```python
from build123d import *

# Parameters (mm, degrees)
F0_R     = 3.175
F1_DEPTH = 57.5
F2_R     = 5
F2_R_2   = 3.175
F3_DEPTH = 5
F4_R     = 4.99999


# Not quite as in the source:
# - a fillet or chamfer is up to 0.001 mm smaller than in the source, because OpenCascade refuses the exact size


with BuildPart() as f1:
    # F0 (on Top) → F1 (new body)
    with BuildSketch(Plane.XY):
        Circle(F0_R)
    extrude(amount=F1_DEPTH)

    # F2 (on face) → F3 (join)
    with BuildSketch(Plane.XY.offset(57.5)):
        Circle(F2_R)
        Circle(F2_R_2, mode=Mode.SUBTRACT)
        Circle(F2_R_2)
    extrude(amount=F3_DEPTH)

    # F4 (radius 5 in the source; OpenCascade refuses exactly that, so slightly less here)
    f4_edges = [f1.edges().sort_by_distance(p)[0] for p in [
        (-5, 0, 62.5),
    ]]
    fillet(f4_edges, radius=F4_R)


solid = f1.part
```
Can you work these out from the model? Positions are in its coordinate system, mm. A direction names the side the tool comes from. Coordinates: 2 decimals unless noted, no trailing zeros. Write each loop counter-clockwise with the first axis right and the second up, starting at its lowest first coordinate (ties: lowest second). Pieces come first, ordered by that corner, then holes. Notation, with made-up numbers: M 61.5,-15.75 L 110.5,-15.75 A18 cw 110.5,18.25 Z; hole C -11.75,-21.75 d10. An arc over 180 degrees is marked long. Write item = value, one per line. Start each with the question number.
Q1. I'm going to push flat-ended pins straight in: pin 1 (1 mm diameter, centred on x = 3.5, y = 0, fed in from +Z); pin 2 (3 mm diameter, centred on x = 0.5, z = 8, fed in from -Y) (3 decimals); pin 3 (1.5 mm diameter, centred on x = 2, z = 28.5, fed in from -Y). Where does each tip first touch, or does it pass through?
Q2. On a 3-axis mill with a long thin cutter (end or side, diameter ignored), from which of +Z, -Z, +X, -X, +Y, -Y can I reach the whole of each face in a straight line? I mean faces 1 (the face through (1, -3.3, 57.5)), 2 (the face through (0, 0, 0)). Say none if no direction works.
Q3. If I drill on L1, parallel to Y at x = 0, z = 45 (3 decimals); L2, parallel to Y at x = 1.5, z = 15; L3, parallel to Z at x = -1.25, y = -4, over which ranges is the centre line in solid material (lowest first)? Write a range as [from, to].
Q4. If we section it at A-A, the plane z = 5.5: Write out the boundary of the cut face in (x, y) (3 decimals), then the cut area to 3 significant figures.
Check sheet entries:
q1.pin_1 = 61.5
q1.pin_2 = -3.175
q1.pin_3 = -2.92
q2.face_1 = -Z
q2.face_2 = -Z, +X, -X, +Y, -Y
q3.L1 = [-3.175, 3.175]
q3.L2 = [-2.8, 2.8]
q3.L3 = [57.5, 60.23]
q4.outline = C 0,0 d6.35
q4.area = 31.7 mm²
